from build123d import *

# Parameters (mm, degrees)
SKIZZE1_R                       = 3.925
AUFSATZ_LINEAR_AUSTRAGEN1_DEPTH = 12
SKIZZE2_R                       = 6
AUFSATZ_LINEAR_AUSTRAGEN2_DEPTH = 6
SKIZZE3_R                       = 19.098593171
AUFSATZ_LINEAR_AUSTRAGEN3_DEPTH = 20
SKIZZE4_R                       = 6.075
SCHNITT_LINEAR_AUSTRAGEN1_DEPTH = 10
VERRUNDUNG1_R                   = 1
AUFSATZ_LINEAR_START            = -20
AUFSATZ_LINEAR_AUSTRAGEN4_DEPTH = 20
VERRUNDUNG2_R                   = 1
KREISMUSTER1_COUNT              = 8
VERRUNDUNG2_OF_KREISMUSTER1_R   = 1
SKIZZE6_R                       = 2.925
AUFSATZ_LINEAR_AUSTRAGEN5_DEPTH = 3.8


with BuildPart() as part:
    # Skizze1 → Aufsatz-Linear austragen1 (new body)
    with BuildSketch(Plane.XY):
        Circle(SKIZZE1_R)
    extrude(amount=AUFSATZ_LINEAR_AUSTRAGEN1_DEPTH)

    # Skizze2 → Aufsatz-Linear austragen2 (add)
    with BuildSketch(Plane(origin=(0, 0, 0), x_dir=(-1, 0, 0), z_dir=(0, 0, -1))):
        Circle(SKIZZE2_R)
    extrude(amount=AUFSATZ_LINEAR_AUSTRAGEN2_DEPTH)

    # Skizze3 → Aufsatz-Linear austragen3 (add)
    with BuildSketch(Plane(origin=(0, 0, -6), x_dir=(-1, 0, 0), z_dir=(0, 0, -1))):
        Circle(SKIZZE3_R)
    extrude(amount=AUFSATZ_LINEAR_AUSTRAGEN3_DEPTH)

    # Skizze4 → Schnitt-Linear austragen1 (cut)
    with BuildSketch(Plane(origin=(0, 0, -26), x_dir=(-1, 0, 0), z_dir=(0, 0, -1))):
        Circle(SKIZZE4_R)
    extrude(amount=-SCHNITT_LINEAR_AUSTRAGEN1_DEPTH, mode=Mode.SUBTRACT)

    # Verrundung1
    verrundung1_edges = [part.edges().sort_by_distance(p)[0] for p in [
        (6.075, 0, -26),
    ]]
    fillet(verrundung1_edges, radius=VERRUNDUNG1_R)

    # Skizze5 → Aufsatz-Linear austragen4 (add)
    with BuildSketch(Plane(origin=(0, 0, -26), x_dir=(-1, 0, 0), z_dir=(0, 0, -1)).offset(AUFSATZ_LINEAR_START)):
        with BuildLine():
            Line((0, 23.039597189), (0, 19.098593171))
            ThreePointArc((0, 19.098593171), (0.750579863, 19.083838476), (1.5, 19.039597189))
            Line((1.5, 19.039597189), (1.5, 23.039597189))
            Line((1.5, 23.039597189), (0, 23.039597189))
        make_face()
        with BuildLine():
            ThreePointArc((-1.5, 19.039597189), (-0.750579863, 19.083838476), (0, 19.098593171))
            Line((0, 19.098593171), (0, 23.039597189))
            Line((0, 23.039597189), (-1.5, 23.039597189))
            Line((-1.5, 23.039597189), (-1.5, 19.039597189))
        make_face()
    aufsatz_linear_austragen4 = extrude(amount=AUFSATZ_LINEAR_AUSTRAGEN4_DEPTH)

    # Verrundung2
    verrundung2_edges = [part.edges().sort_by_distance(p)[0] for p in [
        (-1.5, 23.039597189, -16),
        (0, 23.039597189, -6),
        (1.5, 23.039597189, -16),
        (0, 23.039597189, -26),
    ]]
    fillet(verrundung2_edges, radius=VERRUNDUNG2_R)

    # Kreismuster1: Aufsatz-Linear austragen4 ×8 about axis
    kreismuster1_axis = Axis((0, 0, 0), (0, 0, 1))
    for i in range(1, KREISMUSTER1_COUNT):
        add(aufsatz_linear_austragen4.rotate(kreismuster1_axis, i * 360 / KREISMUSTER1_COUNT))

    # Verrundung2 of Kreismuster1
    verrundung2_of_kreismuster1_edges = [part.edges().sort_by_distance(p)[0] for p in [
        (-17.35211558, 15.230795236, -16),
        (-16.291455408, 16.291455408, -6),
        (-15.230795236, 17.35211558, -16),
        (-16.291455408, 16.291455408, -26),
        (-23.039597189, -1.5, -16),
        (-23.039597189, 0, -6),
        (-23.039597189, 1.5, -16),
        (-23.039597189, 0, -26),
        (-15.230795236, -17.35211558, -16),
        (-16.291455408, -16.291455408, -6),
        (-17.35211558, -15.230795236, -16),
        (-16.291455408, -16.291455408, -26),
        (1.5, -23.039597189, -16),
        (0, -23.039597189, -6),
        (-1.5, -23.039597189, -16),
        (0, -23.039597189, -26),
        (17.35211558, -15.230795236, -16),
        (16.291455408, -16.291455408, -6),
        (15.230795236, -17.35211558, -16),
        (16.291455408, -16.291455408, -26),
        (23.039597189, 1.5, -16),
        (23.039597189, 0, -6),
        (23.039597189, -1.5, -16),
        (23.039597189, 0, -26),
        (15.230795236, 17.35211558, -16),
        (16.291455408, 16.291455408, -6),
        (17.35211558, 15.230795236, -16),
        (16.291455408, 16.291455408, -26),
    ]]
    fillet(verrundung2_of_kreismuster1_edges, radius=VERRUNDUNG2_OF_KREISMUSTER1_R)

    # Skizze6 → Aufsatz-Linear austragen5 (add)
    with BuildSketch(Plane.XY.offset(12)):
        with Locations(Location((0, 0, 0), (0, 0, 180))):
            Circle(SKIZZE6_R)
    extrude(amount=AUFSATZ_LINEAR_AUSTRAGEN5_DEPTH)


solid = part.part
Model file for the job. Use its own axes, mm. A direction names the side the tool comes from. Round coordinates to 2 decimals unless told otherwise and drop trailing zeros. Order: outer loops, then holes, each group sorted by start corner. A loop starts at its lowest first (then second) coordinate and runs counter-clockwise, first axis right, second up.
(1) Band-saw the part on A-A (z = -4.5). List the corners of the cut face in (x, y).
(2) Pin check, flat tips, straight feed: pin 1 (1.5 mm diameter, centred on x = 20.5, z = -18, fed in from -Y); pin 2 (2.5 mm diameter, centred on y = -21, z = -13.5, fed in from +X); pin 3 (6 mm diameter, centred on x = -9.5, y = -10, fed in from +Z); pin 4 (4 mm diameter, centred on x = 1, y = -5.5, fed in from -Z). Stop position of each tip, or through.
(3) Drill centre lines: line 1 (Y direction, x = 0, z = -20.5) (3 decimals); line 2 (X direction, y = -15.5, z = -15). Where is each one in solid material? Low to high.
(4) Band-saw the part on B-B (y = -20). List the corners of the cut face in (x, z).
(5) Band-saw the part on D-D (z = 9). List the corners of the cut face in (x, y) (3 decimals), then the cut area to 3 significant figures.
(6) Pull direction Y, two halves, no side cores. Call faces 5 (the face through (-1.5, 21, -16)), 6 (the face through (16.938, 15.242, -16.14)), 7 (the face through (15.981, -16.011, -6.187)): released by +Y, released by -Y, zero draft, split by the parting line, or undercut.
(7) Band-saw the part on C-C (x = -10). List the corners of the cut face in (y, z).
(8) 3-axis set-ups, long thin cutter, end or side, ignore diameter. For faces 1 (the face through (13.48, -15.6, -15.86)), 2 (the face through (15.6, 13.48, -15.86)), 3 (the face through (-7.39, 17.61, -15.86)), 4 (the face through (-2.893, 2.653, 5.916)): which of +Z, -Z, +X, -X, +Y, -Y reach the whole face in a straight line?
Verdict:
1. outline: circle Ø12 at (0, 0)
2. pin 1: stops at y = -1.5
2. pin 2: stops at x = 1.5
2. pin 3: stops at z = -6
2. pin 4: stops at z = -26
3. line 1: y = -23.04 to -6.075, 6.075 to 23.04
3. line 2: x = -16.9 to -13.38, -11.16 to 11.16, 13.38 to 16.9
4. outline: (-1.5, -26) - (1.5, -26) - (1.5, -6) - (-1.5, -6) - close
5. outline: circle Ø7.85 at (0, 0)
5. area: 48.4 mm2
6. face 5: zero draft
6. face 6: undercut
6. face 7: released by -Y
7. outline: (-16.27, -26) - (16.27, -26) - (16.27, -6) - (-16.27, -6) - close
8. face 1: +Z, -Z, -Y
8. face 2: +Z, -Z, +X
8. face 3: +Z, -Z, +Y
8. face 4: +Z
